```python
from build123d import *

# Parameters (mm, degrees)
F0_R     = 225
F1_DEPTH = 19
F2_R     = 50
F2_R_2   = 37.5
F3_DEPTH = 53


with BuildPart() as f1:
    # F0 (on Top) → F1 (new body)
    with BuildSketch(Plane.XY):
        Circle(F0_R)
    extrude(amount=F1_DEPTH)

    # F2 (on face) → F3 (cut)
    with BuildSketch(Plane.XY.offset(19)):
        Circle(F2_R)
        with Locations((0, 170)):
            Circle(F2_R_2)
        with Locations((-109.273894, 130.227555)):
            Circle(F2_R_2)
        with Locations((-167.417318, 29.52019)):
            Circle(F2_R_2)
        with Locations((-147.224319, -85)):
            Circle(F2_R_2)
        with Locations((-58.143424, -159.747746)):
            Circle(F2_R_2)
        with Locations((58.143424, -159.747746)):
            Circle(F2_R_2)
        with Locations((147.224319, -85)):
            Circle(F2_R_2)
        with Locations((167.417318, 29.52019)):
            Circle(F2_R_2)
        with Locations((109.273894, 130.227555)):
            Circle(F2_R_2)
    extrude(amount=-F3_DEPTH, mode=Mode.SUBTRACT)


solid = f1.part
```
Check sheet for the modelled part. Datum: model origin and axes. Units: mm. Coordinates: 2 decimals unless noted, no trailing zeros. Loops run counter-clockwise (first coordinate to the right, second up) from the corner with the lowest first, then second, coordinate; pieces in that order, holes last.
1) Material ranges on probe 1 along X at (y, z) = (-103.5, 16); probe 2 along Y at (x, z) = (40, 7); probe 3 along X at (y, z) = (-110.5, 3.5), recorded low to high.
2) Sectioned sample at D-D (y = -78). Record the boundary of the cut face in (x, z), and give its area (3 significant figures).
3) Sectioned sample at B-B (y = 178.5). Record the boundary of the cut face in (x, z), and give its area (3 significant figures).
4) Sectioned sample at A-A (x = 13.5). Record the boundary of the cut face in (y, z).
5) Sectioned sample at C-C (x = 64). Record the boundary of the cut face in (y, z).
6) Release check for a two-part mould opening along Y. For faces 1 (the face through (47, -47, 0)), 2 (the face through (-224.782, 9.893, 9.367)), 3 (the face through (-87.9, -182.57, 9.63)), 4 (the face through (203.186, 40.784, 9.633)) record: released by +Y, released by -Y, zero draft, split by the parting line, or undercut.
7) Gauge pin test, flat ends, axial feed: pin 1 (1 mm diameter, centred on x = 41.5, z = 12, fed in from -Y); pin 2 (2 mm diameter, centred on x = -138, z = 3.5, fed in from +Y); pin 3 (10 mm diameter, centred on x = -64, z = 8, fed in from +Y). Record the tip position at first contact, or that the pin passes through.
Check sheet entries:
1. probe 1: x = -199.78 to -179.84, -114.61 to 114.61, 179.84 to 199.78
1. probe 2: y = -221.42 to -192.57, -126.93 to -30, 30 to 221.42
1. probe 3: x = -196 to -174.72, -119.73 to 119.73, 174.72 to 196
2. outline: (-211.05, 0) - (-184.07, 0) - (-184.07, 19) - (-211.05, 19) - close; (-110.38, 0) - (110.38, 0) - (110.38, 19) - (-110.38, 19) - close; (184.07, 0) - (211.05, 0) - (211.05, 19) - (184.07, 19) - close
2. area: 5,220 mm2
3. outline: (-136.98, 0) - (-36.52, 0) - (-36.52, 19) - (-136.98, 19) - close; (36.52, 0) - (136.98, 0) - (136.98, 19) - (36.52, 19) - close
3. area: 3,820 mm2
4. outline: (-224.59, 0) - (-48.14, 0) - (-48.14, 19) - (-224.59, 19) - close; (48.14, 0) - (135.01, 0) - (135.01, 19) - (48.14, 19) - close; (204.99, 0) - (224.59, 0) - (224.59, 19) - (204.99, 19) - close
5. outline: (-215.71, 0) - (-196.79, 0) - (-196.79, 19) - (-215.71, 19) - close; (-122.71, 0) - (215.71, 0) - (215.71, 19) - (-122.71, 19) - close
6. face 1: zero draft
6. face 2: split by the parting line
6. face 3: undercut
6. face 4: undercut
7. pin 1: stops at y = -221.23
7. pin 2: stops at y = 178.48
7. pin 3: stops at y = 217.13
